Work out the finished part from the listing and answer in its coordinate system (mm). A direction names the side the tool comes from. Give positions to 0.01 mm unless a question says otherwise; leave off trailing zeros. Order: outer loops, then holes, each group sorted by start corner. A loop starts at its lowest first (then second) coordinate and runs counter-clockwise, first axis right, second up. Notation, with made-up numbers: (3.25, 14) - (11.25, 14) arc R14 cw to (11.25, 38) - close; hole circle Ø7 at (-15.75, 86). An arc over 180 degrees is marked (long way). Put each result on its own line as item: value.
```python
from build123d import *

# Parameters (mm, degrees)
F1_DEPTH = 558.8
F0_W     = 19.05
F0_H     = 1638.3
F2_DEPTH = 419.1
F3_DEPTH = 558.8
F0_W_2   = 914.4
F0_H_2   = 38.1
F4_DEPTH = 19.05


with BuildPart() as f1:
    # F0 (on Front) → F1 (new body)
    with BuildSketch(Plane.XZ):
        Polygon((0, 120.65), (0, 101.6), (50.8, 101.6), (965.2, 101.6), (1016, 101.6), (1016, 120.65), (996.95, 120.65), (19.05, 120.65), align=None)
    extrude(amount=F1_DEPTH)

    # F0 (on Front) → F2 (join)
    with BuildSketch(Plane.XZ):
        with Locations((1006.475, 939.8)):
            Rectangle(F0_W, F0_H)
        with Locations((9.525, 939.8)):
            Rectangle(F0_W, F0_H)
    extrude(amount=F2_DEPTH)

    # F0 (on Front) → F3 (join)
    with BuildSketch(Plane.XZ):
        Polygon((0, 1778), (0, 1758.95), (19.05, 1758.95), (996.95, 1758.95), (1016, 1758.95), (1016, 1778), align=None)
    extrude(amount=F3_DEPTH)

    # F0 (on Front) → F4 (join)
    with BuildSketch(Plane.XZ):
        with Locations((508, 82.55)):
            Rectangle(F0_W_2, F0_H_2)
    extrude(amount=F4_DEPTH)


solid = f1.part
```
(1) Straight lines are drawn through the part: line 1 (Z direction, x = 710.5, y = -145.5); line 2 (X direction, y = -99, z = 952). For each, find the intervals that lie inside material, in ascending order.
Geometry check:
line 1: z = 101.6 to 120.65, 1758.95 to 1778
line 2: x = 0 to 19.05, 996.95 to 1016
(2) A tool of negligible diameter and unlimited length cuts with its end or side. For faces 1 (the face through (996.95, -207, 928)), 2 (the face through (502, -19.05, 83)), 3 (the face through (16, 0, 544)), from which of +Z, -Z, +X, -X, +Y, -Y can it reach the whole face along a straight path? Write none if from no direction.
Geometry check:
face 1: +Y, -Y
face 2: -Z, +X, -X, -Y
face 3: +Z, -Z, +X, -X, +Y
(3) Determine the mould class of faces 4 (the face through (19.05, -207, 928)), 5 (the face through (1016, -213, 928)), 6 (the face through (515, -275, 1778)) for opening direction Z: pulls with the +Z half, pulls with the -Z half, needs draft (parallel to the pull), parting line crosses it, or undercut.
Geometry check:
face 4: undercut
face 5: needs draft
face 6: pulls with the +Z half
(4) Section B-B, the plane z = 607 is taken. Write down the section's boundary in (x, y).
Geometry check:
outline: (0, -419.1) - (19.05, -419.1) - (19.05, 0) - (0, 0) - close; (996.95, -419.1) - (1016, -419.1) - (1016, 0) - (996.95, 0) - close
(5) Section C-C, the plane y = -53.5 is taken. Write down the section's boundary in (x, z).
Geometry check:
outline: (0, 101.6) - (1016, 101.6) - (1016, 1778) - (0, 1778) - close; hole (19.05, 120.65) - (996.95, 120.65) - (996.95, 1758.95) - (19.05, 1758.95) - close
(6) Given pin 1 (11.5 mm diameter, centred on x = 581, z = 82.5, fed in from -Y); pin 2 (21 mm diameter, centred on y = -5.5, z = 76.5, fed in from -X); pin 3 (12 mm diameter, centred on x = 761, y = -355, fed in from -Z); pin 4 (6 mm diameter, centred on y = -195, z = 532, fed in from -X), each flat-ended and moving along its own axis, determine where each tip first touches the part or whether it passes through.
Geometry check:
pin 1: stops at y = -19.05
pin 2: stops at x = 50.8
pin 3: stops at z = 101.6
pin 4: stops at x = 0
(7) Section A-A, the plane x = 92 is taken. Write down the section's boundary in (y, z).
Geometry check:
outline: (-558.8, 101.6) - (-19.05, 101.6) - (-19.05, 63.5) - (0, 63.5) - (0, 120.65) - (-558.8, 120.65) - close; (-558.8, 1758.95) - (0, 1758.95) - (0, 1778) - (-558.8, 1778) - close
